```python
from build123d import *

# Parameters (mm, degrees)
F0_R     = 9
F1_DEPTH = 10
F3_R     = 12.5
F4_DEPTH = 65
F5_DEPTH = 35
F7_R     = 30
F8_DEPTH = 5


with BuildPart() as f1:
    # F0 (on Front) → F1 (new body, symmetric)
    with BuildSketch(Plane.XZ):
        with BuildLine():
            Line((-60, -70), (60, -70))
            ThreePointArc((60, -70), (67.0710678119, -67.0710678119), (70, -60))
            Line((70, -60), (70, 60))
            ThreePointArc((70, 60), (67.0710678119, 67.0710678119), (60, 70))
            Line((60, 70), (-60, 70))
            ThreePointArc((-60, 70), (-67.0710678119, 67.0710678119), (-70, 60))
            Line((-70, 60), (-70, -60))
            ThreePointArc((-70, -60), (-67.0710678119, -67.0710678119), (-60, -70))
        make_face()
        with Locations((-55, -55)):
            Circle(F0_R, mode=Mode.SUBTRACT)
        with Locations((55, -55)):
            Circle(F0_R, mode=Mode.SUBTRACT)
        with Locations((-55, 55)):
            Circle(F0_R, mode=Mode.SUBTRACT)
        with Locations((55, 55)):
            Circle(F0_R, mode=Mode.SUBTRACT)
    extrude(amount=F1_DEPTH, both=True)

    # F3 (on Top) → F4 (join, symmetric)
    with BuildSketch(Plane.XY):
        with BuildLine():
            Line((-25, -10), (-25, -40))
            ThreePointArc((-25, -40), (0, -65), (25, -40))
            Line((25, -40), (25, -10))
            Line((25, -10), (-25, -10))
        make_face()
        with Locations((0, -40)):
            Circle(F3_R, mode=Mode.SUBTRACT)
    extrude(amount=F4_DEPTH, both=True)


with BuildPart() as f5:
    # F3 (on Top) → F5 (new body, symmetric)
    with BuildSketch(Plane.XY):
        with BuildLine():
            Line((-25, -10), (-25, -40))
            ThreePointArc((-25, -40), (0, -65), (25, -40))
            Line((25, -40), (25, -10))
            Line((25, -10), (-25, -10))
        make_face()
        with Locations((0, -40)):
            Circle(F3_R, mode=Mode.SUBTRACT)
    extrude(amount=F5_DEPTH, both=True)


with BuildPart() as f1_1:
    add(f1.part)

    # F6: cut F5
    add(f5.part, mode=Mode.SUBTRACT)

    # F7 (on face) → F8 (cut)
    with BuildSketch(Plane(origin=(0, 10, 0), x_dir=(-1, 0, 0), z_dir=(0, 1, 0))):
        Circle(F7_R)
    extrude(amount=-F8_DEPTH, mode=Mode.SUBTRACT)


solid = f1_1.part
```
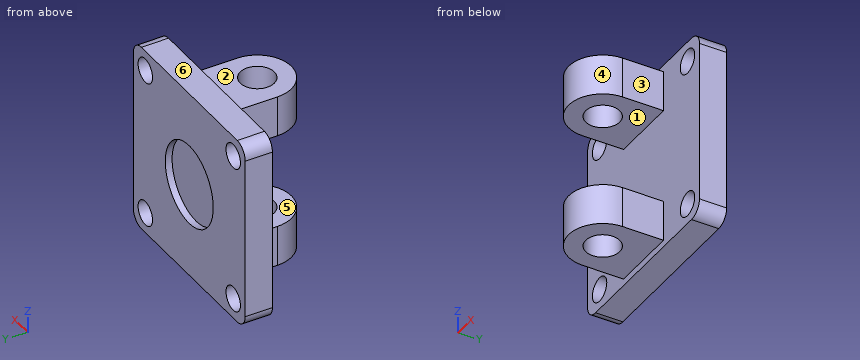
Here's how the part is built. I have some questions about the finished solid (model axes, mm). Face numbers are marked on the shaded views. A direction names the side the tool comes from. Give positions to 0.01 mm unless a question says otherwise; leave off trailing zeros. Write each loop counter-clockwise with the first axis right and the second up, starting at its lowest first coordinate (ties: lowest second). Pieces come first, ordered by that corner, then holes. Notation, with made-up numbers: (12, 65.25) -> (68, 65.25) arc R15 ccw to (68, 84.25) -> close; hole circle Ø8 at (4.25, 71). An arc over 180 degrees is marked (long way). Use one line per item in the form item = value.
1) If I drill on L1, parallel to Z at x = -55, y = -1; L2, parallel to Z at x = -47.5, y = 5.5; L3, parallel to Z at x = 0, y = 8.9, over which ranges is the centre line in solid material (lowest first)? Write a range as [from, to].
Verdict:
L1 = [-70, -64], [-46, 46], [64, 70]
L2 = [-70, -59.97], [-50.03, 50.03], [59.97, 70]
L3 = [-70, -30], [30, 70]
2) Suppose I cut it at D-D (y = -47). Please give me the cut outline in (x, z), and give its area (3 significant figures).
Verdict:
outline = (-24, -65) -> (-10.36, -65) -> (-10.36, -35) -> (-24, -35) -> close; (-24, 35) -> (-10.36, 35) -> (-10.36, 65) -> (-24, 65) -> close; (10.36, -65) -> (24, -65) -> (24, -35) -> (10.36, -35) -> close; (10.36, 35) -> (24, 35) -> (24, 65) -> (10.36, 65) -> close
area = 1,640 mm2
3) On a 3-axis mill with a long thin cutter (end or side, diameter ignored), from which of +Z, -Z, +X, -X, +Y, -Y can I reach the whole of each face in a straight line? I mean the marked faces 1, 2 and 3. Say none if no direction works.
Verdict:
face_1 = +X, -X, -Y
face_2 = +Z, +X, -X, -Y
face_3 = +Z, -Z, +X, -Y
4) Suppose I cut it at B-B (z = -55). Please give me the cut outline in (x, y), and give its area (3 significant figures).
Verdict:
outline = (-70, -10) -> (-64, -10) -> (-64, 10) -> (-70, 10) -> close; (-46, -10) -> (-25, -10) -> (-25, -40) arc R25 ccw to (25, -40) -> (25, -10) -> (46, -10) -> (46, 10) -> (-46, 10) -> close; (64, -10) -> (70, -10) -> (70, 10) -> (64, 10) -> close; hole circle Ø25 at (0, -40)
area = 4,070 mm2
5) I'm going to push flat-ended pins straight in: pin 1 (11 mm diameter, centred on x = -55, z = 55, fed in from -Y) (1 decimal); pin 2 (5 mm diameter, centred on y = -14.5, z = -35.5, fed in from -X); pin 3 (9 mm diameter, centred on y = -19.5, z = -51, fed in from +X); pin 4 (2 mm diameter, centred on x = -18, y = -54.5, fed in from -Z). Where does each tip first touch, or does it pass through?
Verdict:
pin_1 = through
pin_2 = -25
pin_3 = 25
pin_4 = -65
6) Suppose I cut it at A-A (x = -55). Please give me the cut outline in (y, z).
Verdict:
outline = (-10, -70) -> (10, -70) -> (10, -64) -> (-10, -64) -> close; (-10, -46) -> (10, -46) -> (10, 46) -> (-10, 46) -> close; (-10, 64) -> (10, 64) -> (10, 70) -> (-10, 70) -> close
7) We'd pull the mould along Z, two halves only. Please class the marked faces 4, 5 and 6: +Z half, -Z half, draft (parallel to the pull), parting line (faces both ways), or undercut.
Verdict:
face_4 = draft
face_5 = undercut
face_6 = +Z half
8) Suppose I cut it at C-C (y = -24). Please give me the cut outline in (x, z), and give its area (3 significant figures).
Verdict:
outline = (-25, -65) -> (25, -65) -> (25, -35) -> (-25, -35) -> close; (-25, 35) -> (25, 35) -> (25, 65) -> (-25, 65) -> close
area = 3,000 mm2
